The model under review builds one solid part; all positions refer to its coordinate system, in mm. A direction names the side the tool comes from. Round coordinates to 2 decimals unless told otherwise and drop trailing zeros. Order: outer loops, then holes, each group sorted by start corner. A loop starts at its lowest first (then second) coordinate and runs counter-clockwise, first axis right, second up. Notation, with made-up numbers: (-30.75, -30) -> (-2.75, -30) arc R13 cw to (-2.75, -9) -> close; hole circle Ø7 at (-32, -39.75). An arc over 180 degrees is marked (long way). Use a Markdown table: item, result. Add a question column.
```python
from build123d import *

# Parameters (mm, degrees)
F1_DEPTH        = 15
F3_DEPTH        = 8
F4_R            = 3.25
F5_DEPTH        = 22.001
F6_W            = 10
F6_H            = 20.0000007821
F7_DEPTH        = 60.001
F8_W            = 25
F8_H            = 1
F9_DEPTH        = 15
F10_W           = 1
F10_H           = 6.9999992179
F11_DEPTH       = 25
F13_D           = 3.3
F13_DEPTH       = 15
F13_CBORE_D     = 6.5
F13_CBORE_DEPTH = 3
F13_TIP         = 0.9914200214
F15_D           = 5


with BuildPart() as f1:
    # F0 (on Front) → F1 (new body, symmetric)
    with BuildSketch(Plane.XZ):
        Polygon((-6, 16.0000007821), (-6, 0), (0, 0), (0, 30), (-30, 30), (-30, 20.0000007821), (-10, 20.0000007821), align=None)
        Polygon((0, 30), (0, 0), (6, 0), (6, 16.0000007821), (10, 20.0000007821), (30, 20.0000007821), (30, 30), align=None)
    extrude(amount=F1_DEPTH, both=True)

    # F2 (on face) → F3 (cut)
    with BuildSketch(Plane.XY.offset(30)):
        with BuildLine():
            Line((1.75, 6.2599920128), (-1.75, 6.2599920128))
            ThreePointArc((-1.75, 6.2599920128), (0, -6.5), (1.75, 6.2599920128))
        make_face()
    extrude(amount=-F3_DEPTH, mode=Mode.SUBTRACT)

    # F4 (on face) → F5 (cut, through all)
    with BuildSketch(Plane.XY.offset(22)):
        Circle(F4_R)
    extrude(amount=-F5_DEPTH, mode=Mode.SUBTRACT)

    # F6 (on face) → F7 (cut, through all)
    with BuildSketch(Plane(origin=(-30, 0, 0), x_dir=(0, -1, 0), z_dir=(-1, 0, 0))):
        with Locations((0, 10.0000003911)):
            Rectangle(F6_W, F6_H)
    extrude(amount=-F7_DEPTH, mode=Mode.SUBTRACT)

    # F8 (on face) → F9 (cut)
    with BuildSketch(Plane.XZ.offset(15)):
        with Locations((-17.5, 22.5000007821)):
            Rectangle(F8_W, F8_H)
    extrude(amount=-F9_DEPTH, mode=Mode.SUBTRACT)

    # F10 (on face) → F11 (cut)
    with BuildSketch(Plane(origin=(-30, 0, 0), x_dir=(0, -1, 0), z_dir=(-1, 0, 0))):
        with Locations((0.5, 26.5000003911)):
            Rectangle(F10_W, F10_H)
    extrude(amount=-F11_DEPTH, mode=Mode.SUBTRACT)

    # F13
    with Locations(Plane.XZ.offset(15)):
        with Locations((-26, 26.5)):
            CounterBoreHole(F13_D / 2, F13_CBORE_D / 2, F13_CBORE_DEPTH, depth=F13_DEPTH)
            with Locations((0, 0, -(F13_DEPTH + F13_TIP / 2))):  # 118° drill point
                Cone(0, F13_D / 2, F13_TIP, mode=Mode.SUBTRACT)

    # F15 (through all)
    with Locations(Plane(origin=(-6, 0, 0), x_dir=(0, -1, 0), z_dir=(-1, 0, 0))):
        with Locations((-10, 7), (10, 7)):
            Hole(F15_D / 2)


solid = f1.part
```
Q1. Add section B-B (x = -20). Write out the cut boundary in (y, z), then the cut area to 3 significant figures.
Q2. Add section D-D (x = 24). Write out the cut boundary in (y, z), then the cut area to 3 significant figures.
Q3. Add section C-C (y = -5.75). Write out the cut boundary in (x, z).
Q4. Insertion check: pin 1 (4 mm diameter, centred on x = -22, y = -7.5, fed in from -Z); pin 2 (8 mm diameter, centred on y = -8, z = 7, fed in from +X); pin 3 (0.5 mm diameter, centred on y = -8, z = 22.5, fed in from -X). Each pin has a flat end and moves straight along its axis. Give the tip position at first contact, or say it passes through.
Q5. Add section A-A (z = 14). Write out the cut boundary in (x, y).
Q6. Machinability: for faces 1 (the cylindrical face through (-26.705, -13.521, 23.327)), 2 (the flat face through (0, 5, 10)), 3 (the flat face through (-6, 10, 10)), which of the approach directions +Z, -Z, +X, -X, +Y, -Y give a long, thin tool a straight path to every point of the face, cutting with its end or side? Answer none if there is none.
Q7. Wall thickness on line 1 (Z direction, x = -26, y = -10); line 2 (Z direction, x = -13, y = -6.5); line 3 (Y direction, x = -13.5, z = 25.5): over which ranges is each line inside the solid? List them lowest first. Write a range as [from, to].
Q8. Mouldability with a two-part tool opening along Y and no side actions: class faces 4 (the flat face through (-8, 10, 18)), 5 (the flat face through (-18, 0, 26)), 6 (the flat face through (0, -15, 22)), 7 (the cylindrical face through (-2.579, -1.978, 21.014)) as pulls with the +Y half, pulls with the -Y half, needs draft (parallel to the pull), parting line crosses it, or undercut.
Report:
| question | item | result |
|---|---|---|
| 1 | outline | (-15, 20) -> (15, 20) -> (15, 30) -> (0, 30) -> (0, 22) -> (-15, 22) -> close; (-15, 23) -> (-1, 23) -> (-1, 30) -> (-15, 30) -> close |
| 1 | area | 278 mm² |
| 2 | outline | (-15, 20) -> (15, 20) -> (15, 30) -> (-15, 30) -> close |
| 2 | area | 300 mm² |
| 3 | outline | (-30, 20) -> (-10, 20) -> (-6, 16) -> (-6, 0) -> (6, 0) -> (6, 16) -> (10, 20) -> (30, 20) -> (30, 30) -> (3.03, 30) -> (3.03, 22) -> (-3.03, 22) -> (-3.03, 30) -> (-30, 30) -> (-30, 23) -> (-5, 23) -> (-5, 22) -> (-30, 22) -> close; hole circle Ø3.3 at (-26, 26.5) |
| 4 | pin 1 | stops at z = 20 |
| 4 | pin 2 | stops at x = 6 |
| 4 | pin 3 | stops at x = -5 |
| 5 | outline | (-6, -15) -> (6, -15) -> (6, -5) -> (-6, -5) -> close; (-6, 5) -> (6, 5) -> (6, 15) -> (-6, 15) -> close |
| 6 | face 1 | -Y |
| 6 | face 2 | -Z, +X, -X |
| 6 | face 3 | -Z, -X, +Y, -Y |
| 7 | line 1 | z = [20, 22], [23, 24.85], [28.15, 30] |
| 7 | line 2 | z = [20, 22], [23, 30] |
| 7 | line 3 | y = [-15, -1], [0, 15] |
| 8 | face 4 | needs draft |
| 8 | face 5 | undercut |
| 8 | face 6 | pulls with the -Y half |
| 8 | face 7 | undercut |
